The listing builds one solid part. Answer for the finished solid, in the listing's coordinates (mm). Face numbers are marked on the shaded views. A direction names the side the tool comes from. Coordinates: 2 decimals unless noted, no trailing zeros. Order: outer loops, then holes, each group sorted by start corner. A loop starts at its lowest first (then second) coordinate and runs counter-clockwise, first axis right, second up. Notation, with made-up numbers: (3.5, -38.5) -> (16.5, -38.5) arc R10 cw to (16.5, -24.5) -> close; hole circle Ø1 at (79, 84.25). An arc over 180 degrees is marked (long way). Write item = value, one per line.
from build123d import *

# Parameters (mm, degrees)
F1_DEPTH = 10
F2_W     = 5
F2_H     = 5
F2_W_2   = 112
F2_H_2   = 175.8788333833
F3_DEPTH = 50


with BuildPart() as f1:
    # F0 (on Top) → F1 (new body)
    with BuildSketch(Plane.XY):
        with BuildLine():
            Line((86.2209709888, -31.5977521241), (25.5991927239, -66.5977521241))
            Line((25.5991927239, -66.5977521241), (25.5991927239, -76.5977521241))
            Line((25.5991927239, -76.5977521241), (142.5991927239, -76.5977521241))
            Line((142.5991927239, -76.5977521241), (142.5991927239, 113.4022478759))
            Line((142.5991927239, 113.4022478759), (-96.4008072761, 113.4022478759))
            Line((-96.4008072761, 113.4022478759), (-96.4008072761, -76.5977521241))
            Line((-96.4008072761, -76.5977521241), (20.5991927239, -76.5977521241))
            Line((20.5991927239, -76.5977521241), (20.5991927239, -66.5977521241))
            Line((20.5991927239, -66.5977521241), (-40.022585541, -31.5977521241))
            ThreePointArc((-40.022585541, -31.5977521241), (-40.9554062839, -30.6514148366), (-41.2715508997, -29.3607710507))
            Line((-41.2715508997, -29.3607710507), (-65.1872733153, 36.3471362561))
            ThreePointArc((-65.1872733153, 36.3471362561), (-65.299594413, 36.765427467), (-65.3380360189, 37.1968272921))
            Line((-65.3380360189, 37.1968272921), (-77.5682214131, 106.1255387952))
            Line((-77.5682214131, 106.1255387952), (-72.6441826481, 106.9937796835))
            Line((-72.6441826481, 106.9937796835), (-65.3128655033, 65.4158140463))
            Line((-65.3128655033, 65.4158140463), (-65.4888102114, 106.1387293252))
            Line((-65.4888102114, 106.1387293252), (-60.4888102114, 106.1387293252))
            Line((-60.4888102114, 106.1387293252), (-60.4888102114, 38.0572369727))
            Line((-60.4888102114, 38.0572369727), (-60.1816628514, 37.2021866144))
            Line((-60.1816628514, 37.2021866144), (-41.2458632825, 37.2021866144))
            Line((-41.2458632825, 37.2021866144), (-53.4012357192, 106.1387293252))
            Line((-53.4012357192, 106.1387293252), (-48.4771969541, 107.0069702136))
            Line((-48.4771969541, 107.0069702136), (-41.2458632825, 65.7374164892))
            Line((-41.2458632825, 65.7374164892), (-41.2458632825, 106.9938002617))
            Line((-41.2458632825, 106.9938002617), (-36.2458632825, 106.9938002617))
            Line((-36.2458632825, 106.9938002617), (-36.2458632825, 37.2021866144))
            Line((-36.2458632825, 37.2021866144), (-36.2458632825, -15.5121263044))
            Line((-36.2458632825, -15.5121263044), (-17.0029098654, 38.0572575508))
            Line((-17.0029098654, 38.0572575508), (-29.1582823021, 106.9938002617))
            Line((-29.1582823021, 106.9938002617), (-24.234243537, 107.86204115))
            Line((-24.234243537, 107.86204115), (-17.1207785738, 65.2193512955))
            Line((-17.1207785738, 65.2193512955), (-17.3044467615, 107.5445162737))
            Line((-17.3044467615, 107.5445162737), (-12.3044467615, 107.5445162737))
            Line((-12.3044467615, 107.5445162737), (-12.3044467615, 38.0572575508))
            ThreePointArc((-12.3044467615, 38.0572575508), (-12.1916589309, 37.6363276367), (-12.1536783134, 37.2022071925))
            ThreePointArc((-12.1536783134, 37.2022071925), (-12.1916589309, 36.7680867483), (-12.3044467615, 36.3471568342))
            Line((-12.3044467615, 36.3471568342), (-35.8167873917, -28.2524681259))
            Line((-35.8167873917, -28.2524681259), (-33.772585541, -29.4326886146))
            Line((-33.772585541, -29.4326886146), (20.5991927239, -29.4326886146))
            Line((20.5991927239, -29.4326886146), (2.4818595667, 38.1821192256))
            ThreePointArc((2.4818595667, 38.1821192256), (2.4347721068, 38.3943813555), (2.4063054657, 38.6099320248))
            Line((2.4063054657, 38.6099320248), (-9.7679225036, 107.5445162737))
            Line((-9.7679225036, 107.5445162737), (-4.8438837385, 108.412757162))
            Line((-4.8438837385, 108.412757162), (2.4818595667, 66.8664023398))
            Line((2.4818595667, 66.8664023398), (2.4818595667, 108.0871745944))
            Line((2.4818595667, 108.0871745944), (7.3114886982, 108.0871745944))
            Line((7.3114886982, 108.0871745944), (7.3114886982, 39.4762144511))
            Line((7.3114886982, 39.4762144511), (7.4832083847, 38.8291668384))
            Line((7.4832083847, 38.8291668384), (20.5991927239, 38.8291668384))
            Line((20.5991927239, 38.8291668384), (14.4982907316, 108.5627957048))
            Line((14.4982907316, 108.5627957048), (19.479264222, 108.9985744185))
            Line((19.479264222, 108.9985744185), (23.0991927239, 67.4934753996))
            Line((23.0991927239, 67.4934753996), (26.7191212258, 108.9985744185))
            Line((26.7191212258, 108.9985744185), (31.7000947162, 108.5627957048))
            Line((31.7000947162, 108.5627957048), (25.5991927239, 38.8291668384))
            Line((25.5991927239, 38.8291668384), (25.5991927239, -10.5924605114))
            Line((25.5991927239, -10.5924605114), (38.8868967496, 39.4762144511))
            Line((38.8868967496, 39.4762144511), (38.8868967496, 108.0871745944))
            Line((38.8868967496, 108.0871745944), (43.8868967496, 108.0871745944))
            Line((43.8868967496, 108.0871745944), (43.7874143185, 67.2684306459))
            Line((43.7874143185, 67.2684306459), (51.0422691863, 108.412757162))
            Line((51.0422691863, 108.412757162), (55.9663079514, 107.5445162737))
            Line((55.9663079514, 107.5445162737), (43.7920799821, 38.6099320248))
            ThreePointArc((43.7920799821, 38.6099320248), (43.763613341, 38.3943813555), (43.7165258811, 38.1821192256))
            Line((43.7165258811, 38.1821192256), (25.5991927239, -29.4326886146))
            Line((25.5991927239, -29.4326886146), (25.5991927239, -60.8242494322))
            Line((25.5991927239, -60.8242494322), (82.0211007138, -28.249045666))
            Line((82.0211007138, -28.249045666), (58.5309586011, 36.2895893685))
            ThreePointArc((58.5309586011, 36.2895893685), (58.3815477723, 37.2270184447), (58.5923799556, 38.1525705281))
            Line((58.5923799556, 38.1525705281), (60.8801901531, 107.5445162737))
            Line((60.8801901531, 107.5445162737), (65.8774749146, 107.379758838))
            Line((65.8774749146, 107.379758838), (64.5387270896, 72.304022517))
            Line((64.5387270896, 72.304022517), (70.4607553767, 107.8044736843))
            Line((70.4607553767, 107.8044736843), (75.3847941417, 106.936232796))
            Line((75.3847941417, 106.936232796), (63.229421705, 37.9996900851))
            Line((63.229421705, 37.9996900851), (63.536569065, 37.1446397268))
            Line((63.536569065, 37.1446397268), (82.4723686339, 37.1446397268))
            Line((82.4723686339, 37.1446397268), (82.4723686339, 106.936232796))
            Line((82.4723686339, 106.936232796), (87.4723686339, 106.936232796))
            Line((87.4723686339, 106.936232796), (87.4723686339, 65.5010488249))
            Line((87.4723686339, 65.5010488249), (94.6277410706, 106.0811824377))
            Line((94.6277410706, 106.0811824377), (99.5517798357, 105.2129415493))
            Line((99.5517798357, 105.2129415493), (87.4723686339, 37.1446397268))
            Line((87.4723686339, 37.1446397268), (87.4723686339, -15.5696737109))
            Line((87.4723686339, -15.5696737109), (106.7153155628, 37.9996900851))
            Line((106.7153155628, 37.9996900851), (106.7153155628, 105.2129415493))
            Line((106.7153155628, 105.2129415493), (111.7153155628, 105.2129415493))
            Line((111.7153155628, 105.2129415493), (111.5409932174, 65.3674680349))
            Line((111.5409932174, 65.3674680349), (118.8706879995, 106.936232796))
            Line((118.8706879995, 106.936232796), (123.7947267645, 106.0679919077))
            Line((123.7947267645, 106.0679919077), (111.5645413703, 37.1392804046))
            ThreePointArc((111.5645413703, 37.1392804046), (111.5260997644, 36.7078805795), (111.4137786667, 36.2895893685))
            Line((111.4137786667, 36.2895893685), (87.4723686339, -29.4888940865))
            Line((87.4723686339, -29.4888940865), (87.4704533123, -29.4835621298))
            ThreePointArc((87.4704533123, -29.4835621298), (87.1232033779, -30.7046539221), (86.2209709888, -31.5977521241))
        make_face()
        Polygon((-33.772585541, -29.4326886146), (20.5991927239, -60.8242494322), (20.5991927239, -29.4326886146), align=None)
        Polygon((-60.1816628514, 37.2021866144), (-41.2458632825, -15.5121268233), (-41.2458632825, 37.2021866144), align=None)
        Polygon((7.4832083847, 38.8291668384), (20.5991927239, -10.5924605114), (20.5991927239, 38.8291668384), align=None)
        Polygon((63.536569065, 37.1446397268), (82.4723686339, -15.5696737109), (82.4723686339, 37.1446397268), align=None)
    extrude(amount=F1_DEPTH)

    # F2 (on face) → F3 (join)
    with BuildSketch(Plane.XY.offset(10)):
        with Locations((23.0991927239, -74.0977521241)):
            Rectangle(F2_W, F2_H)
        Polygon((25.5991927239, -71.5977521241), (25.5991927239, -76.5977521241), (142.5991927239, -76.5977521241), (142.5991927239, -67.4765855074), (137.5991927239, -67.4765855074), (137.5991927239, -71.5977521241), align=None)
        with Locations((-35.4008072761, -74.0977521241)):
            Rectangle(F2_W_2, F2_H)
        Polygon((-96.4008072761, 113.4022478759), (-96.4008072761, -76.5977521241), (-91.4008072761, -76.5977521241), (-91.4008072761, -71.5977521241), (-91.4008072761, 108.4022478759), (-91.4008072761, 113.4022478759), align=None)
        with Locations((140.0991927239, 20.4628311843)):
            Rectangle(F2_W, F2_H_2)
        Polygon((142.5991927239, 113.4022478759), (-91.4008072761, 113.4022478759), (-91.4008072761, 108.4022478759), (-4.9034848615, 108.4022478759), (-4.8438837385, 108.412757162), (-4.8420306678, 108.4022478759), (14.5123368465, 108.4022478759), (14.4982907316, 108.5627957048), (19.479264222, 108.9985744185), (19.531273722, 108.4022478759), (26.6671117258, 108.4022478759), (26.7191212258, 108.9985744185), (31.7000947162, 108.5627957048), (31.6860486013, 108.4022478759), (51.0404161156, 108.4022478759), (51.0422691863, 108.412757162), (51.1018703093, 108.4022478759), (137.5991927239, 108.4022478759), (142.5991927239, 108.4022478759), align=None)
    extrude(amount=F3_DEPTH)


solid = f1.part
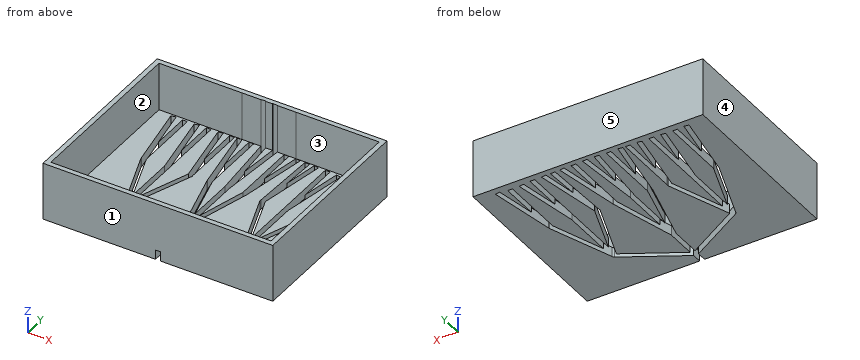
Q1. A tool of negligible diameter and unlimited length cuts with its end or side. For the marked faces 1 and 2, from which of +Z, -Z, +X, -X, +Y, -Y can it reach the whole face along a straight path? Write none if from no direction.
The answers:
face_1 = +Z, -Z, +X, -X, -Y
face_2 = +Z
Q2. Section B-B, the plane x = -56 is taken. Give the vertices of the cut face in (y, z), plus the area to 3 significant figures.
The answers:
outline = (-76.6, 0) -> (11.11, 0) -> (11.11, 10) -> (-71.6, 10) -> (-71.6, 60) -> (-76.6, 60) -> close; (25.56, 0) -> (113.4, 0) -> (113.4, 60) -> (108.4, 60) -> (108.4, 10) -> (25.56, 10) -> close
area = 2,260 mm2
Q3. Section D-D, the plane x = 47 is taken. Give the vertices of the cut face in (y, z).
The answers:
outline = (-76.6, 0) -> (-54.24, 0) -> (-54.24, 10) -> (-71.6, 10) -> (-71.6, 60) -> (-76.6, 60) -> close; (-48.47, 0) -> (56.77, 0) -> (56.77, 10) -> (-48.47, 10) -> close; (85.49, 0) -> (113.4, 0) -> (113.4, 60) -> (108.4, 60) -> (108.4, 10) -> (85.49, 10) -> close
Q4. Find the intervals of material crossed by line 1 along X through (y, z) = (42.5, 19); line 2 along Y through (x, z) = (46.5, 55.5); line 3 along Z through (x, y) = (44.5, -63), in increasing order.
The answers:
line_1 = -96.4 to -91.4, 137.6 to 142.6
line_2 = -76.6 to -71.6, 108.4 to 113.4
line_3 = 0 to 10
Q5. This flat-tipped pin is pushed along its axis until it touches: pin 1 Ø8 at (x, y) = (-69, 19.5) entering from +Z. Where does it stop, or does it pass through?
The answers:
pin_1 = 10
Q6. The mould has two halves that part along X. Classify the marked faces 3, 4 and 5: released by +X, released by -X, zero draft, split by the parting line, or undercut.
The answers:
face_3 = undercut
face_4 = released by -X
face_5 = zero draft
Q7. Section A-A, the plane y = -54 is taken. Give the vertices of the cut face in (x, z).
The answers:
outline = (-96.4, 0) -> (-1.22, 0) -> (-1.22, 10) -> (-91.4, 10) -> (-91.4, 60) -> (-96.4, 60) -> close; (8.78, 0) -> (20.6, 0) -> (20.6, 10) -> (8.78, 10) -> close; (25.6, 0) -> (37.42, 0) -> (37.42, 10) -> (25.6, 10) -> close; (47.42, 0) -> (142.6, 0) -> (142.6, 60) -> (137.6, 60) -> (137.6, 10) -> (47.42, 10) -> close
